```python
from build123d import *

# Parameters (mm, degrees)
SKETCH1_W          = 50
SKETCH1_H          = 13
EXTRUDE1_DEPTH     = 12.7
SKETCH2_W          = 44.7
SKETCH2_H          = 11
CUT_EXTRUDE1_DEPTH = 11
SKETCH3_R          = 0.5
EXTRUDE2_DEPTH     = 15


with BuildPart() as part:
    # Sketch1 → Extrude1 (new body)
    with BuildSketch(Plane(origin=(0, 0, 0), x_dir=(1, 0, 0), z_dir=(0, 1, 0))):
        Rectangle(SKETCH1_W, SKETCH1_H)
    extrude(amount=EXTRUDE1_DEPTH)

    # Sketch2 → Cut-Extrude1 (cut)
    with BuildSketch(Plane(origin=(0, 12.7, 0), x_dir=(-1, 0, 0), z_dir=(0, 1, 0))):
        Rectangle(SKETCH2_W, SKETCH2_H)
    extrude(amount=-CUT_EXTRUDE1_DEPTH, mode=Mode.SUBTRACT)

    # Sketch3 → Extrude2 (add)
    with BuildSketch(Plane.XZ):
        with Locations(Location((-22.35, 0, 0), (0, 0, 90))):
            Circle(SKETCH3_R)
        with Locations(Location((22.35, 0, 0), (0, 0, 90))):
            Circle(SKETCH3_R)
    extrude(amount=EXTRUDE2_DEPTH)


solid = part.part
```
CAD build for the part. Positions are in the model's coordinates, mm. A direction names the side the tool comes from. Give positions to 0.01 mm unless a question says otherwise; leave off trailing zeros. Write each loop counter-clockwise with the first axis right and the second up, starting at its lowest first coordinate (ties: lowest second). Pieces come first, ordered by that corner, then holes. Notation, with made-up numbers: M 21,-13 L 29,-13 A28 cw 29,5 Z; hole C 44.25,85 d9. An arc over 180 degrees is marked long. Return JSON: item names as keys, results as strings. Group by question number.
(1) Band-saw the part on B-B (z = 4.25). Give the cut face in (x, y).
(2) Drill centre lines: L1, parallel to Z at x = -13.5, y = 8; L2, parallel to X at y = 7.5, z = -1; L3, parallel to Y at x = -22, z = -4.5. Where is each one in solid material? Low to high. Write a range as [from, to].
(3) Flat gauge pin, fed straight in: pin 1 Ø5 at (y, z) = (-7.5, 2) entering from +X. Where does the tip first touch, or does it go through?
(4) Band-saw the part on C-C (y = 9.75). Give the cut face in (x, z), and give its area (3 significant figures).
(5) 3-axis set-ups, long thin cutter, end or side, ignore diameter. For faces 1 (the face through (25, 6, 0)), 2 (the face through (0, 1.7, 0)), 3 (the face through (-21.862, -7.395, -0.108)): which of +Z, -Z, +X, -X, +Y, -Y reach the whole face in a straight line?
(6) Band-saw the part on A-A (x = 2). Give the cut face in (y, z), and give its area (3 significant figures).
(7) Mould opens along X. For faces 4 (the face through (0, 6, 6.5)), 5 (the face through (-22.35, 7, 0)), 6 (the face through (-25, 6, 0)) say: pulls with the +X half, pulls with the -X half, needs draft (parallel to the pull), parting line crosses it, or undercut.
(8) Band-saw the part on D-D (z = 0). Give the cut face in (x, y).
Entries:
{
 "1": {"outline": "M -25,0 L 25,0 L 25,12.7 L 22.35,12.7 L 22.35,1.7 L -22.35,1.7 L -22.35,12.7 L -25,12.7 Z"},
 "2": {"L1": "z = [-6.5, -5.5], [5.5, 6.5]", "L2": "x = [-25, -22.35], [22.35, 25]", "L3": "y = [0, 1.7]"},
 "3": {"pin 1": "stops at x = 22.85"},
 "4": {"outline": "M -25,-6.5 L 25,-6.5 L 25,6.5 L -25,6.5 Z; hole M -22.35,-5.5 L 22.35,-5.5 L 22.35,5.5 L -22.35,5.5 Z", "area": "158 mm^2"},
 "5": {"face 1": "+Z, -Z, +X, +Y, -Y", "face 2": "+Y", "face 3": "-Y"},
 "6": {"outline": "M 0,-6.5 L 12.7,-6.5 L 12.7,-5.5 L 1.7,-5.5 L 1.7,5.5 L 12.7,5.5 L 12.7,6.5 L 0,6.5 Z", "area": "44.1 mm^2"},
 "7": {"face 4": "needs draft", "face 5": "undercut", "face 6": "pulls with the -X half"},
 "8": {"outline": "M -25,0 L -22.85,0 L -22.85,-15 L -21.85,-15 L -21.85,0 L 21.85,0 L 21.85,-15 L 22.85,-15 L 22.85,0 L 25,0 L 25,12.7 L 22.35,12.7 L 22.35,1.7 L -22.35,1.7 L -22.35,12.7 L -25,12.7 Z"}
}
